```python
from build123d import *

# Parameters (mm, degrees)
BOSS_EXTRUDE1_DEPTH         = 22
CUT_EXTRUDE1_DEPTH          = 8
F_1_4_0_25_DIAMETER_HOLE1_D = 6.35
FILLET2_R                   = 1


with BuildPart() as part:
    # Sketch2 → Boss-Extrude1 (new body)
    with BuildSketch(Plane.XY):
        Polygon((0, 0), (18, 0), (14.00115161, 12), (3.99884839, 12), align=None)
    extrude(amount=-BOSS_EXTRUDE1_DEPTH)

    # Sketch3 → Cut-Extrude1 (cut)
    with BuildSketch(Plane.XZ):
        Polygon((13, -13.309401077), (13, -8.690598923), (9, -6.381197846), (5, -8.690598923), (5, -13.309401077), (9, -15.618802154), align=None)
    extrude(amount=-CUT_EXTRUDE1_DEPTH, mode=Mode.SUBTRACT)

    # 1/4 (0.25) Diameter Hole1 (through all)
    with Locations(Plane(origin=(0, 12, 0), x_dir=(1, 0, 0), z_dir=(0, 1, 0))):
        with Locations((8.99884839, 11)):
            Hole(F_1_4_0_25_DIAMETER_HOLE1_D / 2)

    # Fillet2
    fillet2_edges = [part.edges().sort_by_distance(p)[0] for p in [
        (16.000575805, 6, -22),
        (11, 0, -14.464101615),
        (13, 0, -11),
        (11, 0, -7.535898385),
        (7, 0, -7.535898385),
        (5, 0, -11),
        (7, 0, -14.464101615),
        (12.17384839, 12, -11),
        (1.999424195, 6, -22),
        (16.000575805, 6, 0),
        (9, 0, 0),
        (1.999424195, 6, 0),
        (18, 0, -11),
        (0, 0, -11),
        (9, 0, -22),
    ]]
    fillet(fillet2_edges, radius=FILLET2_R)


solid = part.part
```
Geometry: final body of the model. Coordinates: model frame, mm. A direction names the side the tool comes from. Coordinates: 2 decimals unless noted, no trailing zeros. Order: outer loops, then holes, each group sorted by start corner. A loop starts at its lowest first (then second) coordinate and runs counter-clockwise, first axis right, second up. Notation, with made-up numbers: (-8.5, 86) -> (38.5, 86) arc R23 cw to (38.5, 105) -> close; hole circle Ø1 at (7, 71.25). An arc over 180 degrees is marked (long way). Use CSV: the item, a comma, the result in double quotes.
1) Pin query (flat end, axial travel): pin 1 Ø1.4 at (y, z) = (3.5, -10.5) entering from +X; pin 2 Ø8.5 at (x, z) = (9, -11) entering from -Y; pin 3 Ø3.5 at (y, z) = (5, -10) entering from -X. Return the tip coordinate at first contact, or that it passes through.
Findings:
pin 1,"stops at x = 17.07"
pin 2,"stops at y = 0.34"
pin 3,"stops at x = 1.08"
2) Line query: line 1 (Z direction, x = 11.5, y = 7.5); line 2 (X direction, y = 2, z = -14.5); line 3 (X direction, y = 9, z = -11). Output: solid intervals per line, ascending.
Findings:
line 1,"z = -22 to -14.18, -7.82 to 0"
line 2,"x = 0.67 to 7.06, 10.94 to 17.33"
line 3,"x = 3 to 5.82, 12.17 to 15"
3) Section A-A on z = -11. Output: boundary loops of the cut face in (x, y).
Findings:
outline,"(0.44, 1.32) arc R1 ccw to (1.39, 0) -> (4, 0) arc R1 ccw to (5, 1) -> (5, 8) -> (5.82, 8) -> (5.82, 11) arc R1 ccw to (4.82, 12) -> (4, 12) -> close; (12.17, 8) -> (13, 8) -> (13, 1) arc R1 ccw to (14, 0) -> (16.61, 0) arc R1 ccw to (17.56, 1.32) -> (14, 12) -> (13.17, 12) arc R1 ccw to (12.17, 11) -> close"
4) Section B-B on z = -17.75. Output: boundary loops of the cut face in (x, y).
Findings:
outline,"(0.44, 1.32) arc R1 ccw to (1.39, 0) -> (16.61, 0) arc R1 ccw to (17.56, 1.32) -> (14, 12) -> (4, 12) -> close"
5) Access query for faces 4 (the cylindrical face through (15.42, 6.8, -21.71)), 5 (the flat face through (5, 4, -11)). Directions: +Z, -Z, +X, -X, +Y, -Y. A direction counts if a zero-diameter tool reaches every point of the face in a straight line with its end or side. Return the directions, or none.
Findings:
face 4,"-Z, +X, +Y"
face 5,"-Y"
6) Mould query, pull axis Z, two halves, no side actions, for faces 1 (the cylindrical face through (9.107, 0.285, -0.301)), 2 (the flat face through (10.97, 4.45, -14.48)), 3 (the flat face through (3.8, 0, -10.9)). Classes: +Z half, -Z half, draft (parallel to the pull), parting line (faces both ways), or undercut.
Findings:
face 1,"+Z half"
face 2,"undercut"
face 3,"draft"
